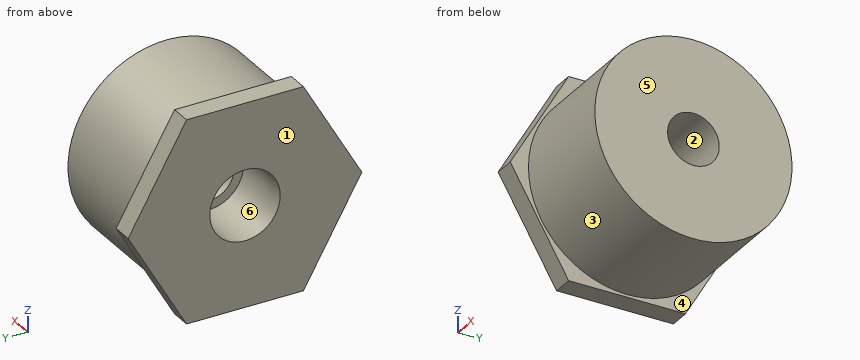
from build123d import *

# Parameters (mm, degrees)
SKETCH2_R           = 10.7696
BOSS_EXTRUDE1_DEPTH = 6.35


with BuildPart() as part:
    # Sketch1 → Revolve1 (revolve)
    with BuildSketch(Plane.XY):
        Polygon((-41.275, -30.1625), (0, -30.1625), (0, -7.8994), (-22.225, -7.8994), (-22.225, -10.6172), (-41.275, -10.7696), align=None)
    revolve(axis=Axis((-41.275, 0, 0), (1, 0, 0)))

    # Sketch2 → Boss-Extrude1 (add)
    with BuildSketch(Plane.ZY.offset(41.275)):
        Polygon((0, 35.745198541), (-30.95625, 17.872599271), (-30.95625, -17.872599271), (0, -35.745198541), (30.95625, -17.872599271), (30.95625, 17.872599271), align=None)
        Circle(SKETCH2_R, mode=Mode.SUBTRACT)
    extrude(amount=-BOSS_EXTRUDE1_DEPTH)


solid = part.part
Verification items for the finished model (mm, model axes). Face numbers are marked on the shaded views. A direction names the side the tool comes from. Give positions to 0.01 mm unless a question says otherwise; leave off trailing zeros. Loops run counter-clockwise (first coordinate to the right, second up) from the corner with the lowest first, then second, coordinate; pieces in that order, holes last.
1. Tool access check on the marked faces 4, 5 and 6. Record the directions out of +Z, -Z, +X, -X, +Y, -Y that give a thin tool (end or side, any length) a straight path to the whole face; none if there is none.
Derived:
face 4: +X
face 5: +Z, -Z, +X, +Y, -Y
face 6: -X
2. Cross-section at A-A on x = -11. Record the cut outline in (y, z) (1 decimal), and give its area (3 significant figures).
Derived:
outline: circle Ø60.3 at (0, 0); hole circle Ø15.8 at (0, 0)
area: 2,660 mm2
3. Go/stop test with flat-tipped pins: P1, Ø17, axis at y = -3.5, z = -3, coming from the -X side (3 decimals); P2, Ø2, axis at x = -6.5, y = 16.5, coming from the -Z side; P3, Ø5, axis at x = -21.5, y = 11, coming from the +Z side; P4, Ø3, axis at x = -34.5, z = -3.5, coming from the -Y side (3 decimals). Record where each tip stops, or that it passes through.
Derived:
P1: stops at x = -41.275
P2: stops at z = -25.88
P3: stops at z = 28.94
P4: stops at y = -34.555
4. Cross-section at C-C on y = -24.5. Record the cut outline in (x, z) (3 decimals), and give its area (3 significant figures).
Derived:
outline: (-41.275, -19.477) - (-34.925, -19.477) - (-34.925, -17.593) - (0, -17.593) - (0, 17.593) - (-34.925, 17.593) - (-34.925, 19.477) - (-41.275, 19.477) - close
area: 1,480 mm2
5. Material ranges on probe 1 along Z at (x, y) = (-13, 0); probe 2 along X at (y, z) = (9.5, 1) (3 decimals), recorded low to high.
Derived:
probe 1: z = -30.16 to -7.9, 7.9 to 30.16
probe 2: x = -22.225 to 0
6. Release check for a two-part mould opening along Y. For the marked faces 1, 2 and 3 record: +Y half, -Y half, draft (parallel to the pull), parting line (faces both ways), or undercut.
Derived:
face 1: draft
face 2: undercut
face 3: parting line
7. Cross-section at B-B on z = -24. Record the cut outline in (x, y) (3 decimals), and give its area (3 significant figures).
Derived:
outline: (-41.275, -21.889) - (-34.925, -21.889) - (-34.925, -18.27) - (0, -18.27) - (0, 18.27) - (-34.925, 18.27) - (-34.925, 21.889) - (-41.275, 21.889) - close
area: 1,550 mm2
